```python
from build123d import *

# Parameters (mm, degrees)
F0_R      = 7
F1_DEPTH  = 16
F4_DEPTH  = 1
F5_R      = 4
F6_DEPTH  = 14
F8_DEPTH  = 16.001
F10_DEPTH = 15.001
F12_DEPTH = 15.002


with BuildPart() as f1:
    # F0 (on Top) → F1 (new body)
    with BuildSketch(Plane.XY):
        Circle(F0_R)
    extrude(amount=F1_DEPTH)

    # F3 (on offset) → F4 (join)
    with BuildSketch(Plane.XY.offset(15)):
        Polygon((8.8388347648, 8.8388347648), (0, 12.5), (-8.8388347648, 8.8388347648), (-12.5, 0), (-8.8388347648, -8.8388347648), (0, -12.5), (8.8388347648, -8.8388347648), (12.5, 0), align=None)
    extrude(amount=-F4_DEPTH)

    # F5 (on Top) → F6 (cut, through all)
    with BuildSketch(Plane.XY):
        Circle(F5_R)
    extrude(amount=F6_DEPTH, mode=Mode.SUBTRACT)

    # F7 (on face) → F8 (cut, through all)
    with BuildSketch(Plane.XY.offset(16)):
        with BuildLine():
            Line((-2, 1.5), (-2, -1.5))
            ThreePointArc((-2, -1.5), (0, -2.5), (2, -1.5))
            Line((2, -1.5), (2, 1.5))
            ThreePointArc((2, 1.5), (0, 2.5), (-2, 1.5))
        make_face()
    extrude(amount=-F8_DEPTH, mode=Mode.SUBTRACT)


with BuildPart() as f10:
    # F9 (on face) → F10 (new body, through all)
    with BuildSketch(Plane.XY.offset(15)):
        with BuildLine():
            Line((0, 12.5), (-8.8388347648, 8.8388347648))
            ThreePointArc((-8.8388347648, 8.8388347648), (-3.9531824429, 9.5438266683), (0, 12.5))
        make_face()
    extrude(amount=-F10_DEPTH)


with BuildPart() as f12_tool:
    # F11 (on face) → F12 (new body, through all)
    with BuildSketch(Plane.XY.offset(15)):
        with BuildLine():
            ThreePointArc((-8.8388347648, 8.8388347648), (-3.9531824429, 9.5438266683), (0, 12.5))
            Line((0, 12.5), (-8.8388347648, 8.8388347648))
        make_face()
    extrude(amount=-F12_DEPTH)


with BuildPart() as f1_1:
    add(f1.part)

    # F12: cut by f12_tool
    add(f12_tool.part, mode=Mode.SUBTRACT)


with BuildPart() as f10_1:
    add(f10.part)

    # F12: cut by f12_tool
    add(f12_tool.part, mode=Mode.SUBTRACT)


solid = f1_1.part
```
Model file for the job. Use its own axes, mm. A direction names the side the tool comes from. Round coordinates to 2 decimals unless told otherwise and drop trailing zeros. Loops run counter-clockwise (first coordinate to the right, second up) from the corner with the lowest first, then second, coordinate; pieces in that order, holes last. Notation, with made-up numbers: M 70.5,54.25 L 129.5,54.25 A17 cw 129.5,64.25 Z; hole C 36.5,-15 d2. An arc over 180 degrees is marked long. Put each result on its own line as item: value. Start each with the question number.
Item 1: Cut at A-A (z = 14.5). List the corners of the cut face in (x, y), then the cut area to 3 significant figures.
Item 2: Cut at C-C (y = -2). List the corners of the cut face in (x, z).
Item 3: Drill centre lines: line 1 along Y through (x, z) = (0, 3.75); line 2 along Z through (x, y) = (3, 8.25); line 3 along Y through (x, z) = (2.25, 12.5). Where is each one in solid material? Low to high.
Item 4: 3-axis set-ups, long thin cutter, end or side, ignore diameter. For faces 5 (the face through (6.466, -2.681, 6.902)), 6 (the face through (10.644, -4.481, 14.507)), 7 (the face through (2, 0, 15)), 8 (the face through (5.4, -5.4, 15)): which of +Z, -Z, +X, -X, +Y, -Y reach the whole face in a straight line?
Item 5: Cut at D-D (x = 6). List the corners of the cut face in (y, z).
Item 6: Cut at B-B (x = 1). List the corners of the cut face in (y, z), then the cut area to 3 significant figures.
Item 7: Mould opens along X. For faces 1 (the face through (-2, 0, 15)), 2 (the face through (0, -3, 16)), 3 (the face through (-4.018, 9.517, 14.507)), 4 (the face through (6.466, -2.681, 15.493)) say: released by +X, released by -X, zero draft, split by the parting line, or undercut.
Item 8: Drop flat-ended pins along their axis: P1, Ø8, axis at x = 6, z = 6, coming from the +Y side; P2, Ø7, axis at x = 0, y = 0, coming from the -Z side; P3, Ø4, axis at y = -3, z = 12.5, coming from the +X side. Give the stop position or say it passes through.
Answer block:
1. outline: M -12.5,0 L -8.84,-8.84 L 0,-12.5 L 8.84,-8.84 L 12.5,0 L 8.84,8.84 L 0,12.5 A10 cw -8.84,8.84 Z; hole M -2,-1.5 A2.5 ccw 2,-1.5 L 2,1.5 A2.5 ccw -2,1.5 Z
1. area: 416 mm2
2. outline: M -11.67,14 L -6.71,14 L -6.71,0 L -3.46,0 L -3.46,14 L -1.5,14 L -1.5,16 L -6.71,16 L -6.71,15 L -11.67,15 Z; M 1.5,14 L 3.46,14 L 3.46,0 L 6.71,0 L 6.71,14 L 11.67,14 L 11.67,15 L 6.71,15 L 6.71,16 L 1.5,16 Z
3. line 1: -7 to -4, 4 to 7
3. line 2: 14 to 15
3. line 3: -6.63 to -3.31, 3.31 to 6.63
4. face 5: -Z
4. face 6: +Z, -Z, +X, -Y
4. face 7: +Z, -Z
4. face 8: +Z
5. outline: M -10.01,14 L -3.61,14 L -3.61,0 L 3.61,0 L 3.61,14 L 10.01,14 L 10.01,15 L 3.61,15 L 3.61,16 L -3.61,16 L -3.61,15 L -10.01,15 Z
6. outline: M -12.09,14 L -6.93,14 L -6.93,0 L -3.87,0 L -3.87,14 L -2.29,14 L -2.29,16 L -6.93,16 L -6.93,15 L -12.09,15 Z; M 2.29,14 L 3.87,14 L 3.87,0 L 6.93,0 L 6.93,14 L 12.09,14 L 12.09,15 L 6.93,15 L 6.93,16 L 2.29,16 Z
6. area: 114 mm2
7. face 1: undercut
7. face 2: zero draft
7. face 3: undercut
7. face 4: split by the parting line
8. P1: y = 6.71
8. P2: z = 14
8. P3: x = 11.81
